```python
from build123d import *

# Parameters (mm, degrees)
PROFILE_SKETCH_W      = 990.6
PROFILE_SKETCH_H      = 304.8
PROFILE_EXTRUDE_DEPTH = 25.4
EDGE_CHAMFER_SIZE     = 12.7


with BuildPart() as part:
    # Profile Sketch → Profile Extrude (new body)
    with BuildSketch(Plane.XY):
        Rectangle(PROFILE_SKETCH_W, PROFILE_SKETCH_H)
    extrude(amount=PROFILE_EXTRUDE_DEPTH)

    # Edge Chamfer
    edge_chamfer_edges = [part.edges().sort_by_distance(p)[0] for p in [
        (-495.3, 0, 25.4),
        (0, -152.4, 25.4),
        (495.3, 0, 25.4),
        (0, 152.4, 25.4),
    ]]
    chamfer(edge_chamfer_edges, length=EDGE_CHAMFER_SIZE)


solid = part.part
```
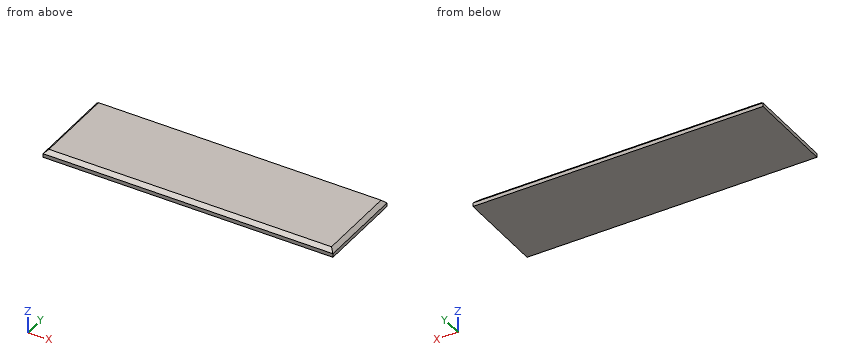
The listing builds one solid part. Answer for the finished solid, in the listing's coordinates (mm). Coordinates: 2 decimals unless noted, no trailing zeros. Order: outer loops, then holes, each group sorted by start corner. A loop starts at its lowest first (then second) coordinate and runs counter-clockwise, first axis right, second up. Notation, with made-up numbers: M 1,77 L 55,77 A9 cw 55,88 Z; hole C 78.5,5 d3. An arc over 180 degrees is marked long. Answer as a JSON object with one key per item and string values. Group by question number.
1. Section A-A on x = -110 is taken. Write down the section's boundary in (y, z).
2. Flat-ended cylindrical pins translate along their axes: P1, Ø10, axis at x = 14.5, z = 20, coming from the -Y side; P2, Ø3, axis at x = -359, z = 21.5, coming from the +Y side; P3, Ø12, axis at x = -246.5, y = 19, coming from the -Z side. Find the tip coordinate at first contact, or state that the pin passes through.
3. Straight lines are drawn through the part: line 1 (X direction, y = -122, z = 24); line 2 (Y direction, x = 68, z = 16.25); line 3 (Y direction, x = 418.5, z = 14). For each, find the intervals that lie inside material, in ascending order.
4. Section B-B on z = 20.25 is taken. Write down the section's boundary in (x, y).
Values follow:
{
 "1": {"outline": "M -152.4,0 L 152.4,0 L 152.4,12.7 L 139.7,25.4 L -139.7,25.4 L -152.4,12.7 Z"},
 "2": {"P1": "y = -150.1", "P2": "y = 145.1", "P3": "z = 0"},
 "3": {"line 1": "-484 to 484", "line 2": "-148.85 to 148.85", "line 3": "-151.1 to 151.1"},
 "4": {"outline": "M -487.75,-144.85 L 487.75,-144.85 L 487.75,144.85 L -487.75,144.85 Z"}
}
